```python
from build123d import *

# Parameters (mm, degrees)
SKETCH1_W           = 50
SKETCH1_H           = 52
BOSS_EXTRUDE1_DEPTH = 82.5
SKETCH2_R           = 15
CUT_EXTRUDE1_DEPTH  = 80
SKETCH3_R           = 5.25
SKETCH3_R_2         = 1.75
CUT_EXTRUDE2_DEPTH  = 91.040268769
SKETCH4_R           = 1.7
CUT_EXTRUDE4_DEPTH  = 100.911210582
SKETCH6_W           = 27.5
SKETCH6_H           = 52
CUT_EXTRUDE5_DEPTH  = 100.911210582
CUT_EXTRUDE6_DEPTH  = 100.911210582
CUT_EXTRUDE7_DEPTH  = 101.673978763
FILLET1_R           = 3


with BuildPart() as part:
    # Sketch1 → Boss-Extrude1 (new body)
    with BuildSketch(Plane.XY):
        Rectangle(SKETCH1_W, SKETCH1_H)
    extrude(amount=BOSS_EXTRUDE1_DEPTH)

    # Sketch2 → Cut-Extrude1 (cut)
    with BuildSketch(Plane(origin=(0, 0, 0), x_dir=(-1, 0, 0), z_dir=(0, 0, -1))):
        Circle(SKETCH2_R)
    extrude(amount=-CUT_EXTRUDE1_DEPTH, mode=Mode.SUBTRACT)

    # Sketch3 → Cut-Extrude2 (cut, through all)
    with BuildSketch(Plane.XY.offset(82.5)):
        Circle(SKETCH3_R)
        with Locations((-8, 0)):
            Circle(SKETCH3_R_2)
        with Locations(Location((8, 0, 0), (0, 0, 180))):
            Circle(SKETCH3_R_2)
    extrude(amount=-CUT_EXTRUDE2_DEPTH, mode=Mode.SUBTRACT)

    # Sketch4 → Cut-Extrude4 (cut, through all)
    with BuildSketch(Plane(origin=(25, 0, 0), x_dir=(0, 0, -1), z_dir=(1, 0, 0))):
        with Locations(Location((-57.5, 20, 0), (0, 0, 90))):
            Circle(SKETCH4_R)
        with Locations(Location((-57.5, -20, 0), (0, 0, 270))):
            Circle(SKETCH4_R)
    extrude(amount=-CUT_EXTRUDE4_DEPTH, mode=Mode.SUBTRACT)

    # Sketch6 → Cut-Extrude5 (cut, through all)
    with BuildSketch(Plane(origin=(25, 0, 0), x_dir=(0, 0, -1), z_dir=(1, 0, 0))):
        with Locations((-13.75, 0)):
            Rectangle(SKETCH6_W, SKETCH6_H)
    extrude(amount=-CUT_EXTRUDE5_DEPTH, mode=Mode.SUBTRACT)

    # Sketch9 → Cut-Extrude6 (cut, through all)
    with BuildSketch(Plane(origin=(25, 0, 0), x_dir=(0, 0, -1), z_dir=(1, 0, 0))):
        Polygon((-82.5, 26), (-82.5, 16), (-67.5, 26), align=None)
        Polygon((-82.5, -16), (-67.5, -26), (-82.5, -26), align=None)
    extrude(amount=-CUT_EXTRUDE6_DEPTH, mode=Mode.SUBTRACT)

    # Sketch10 → Cut-Extrude7 (cut, through all)
    with BuildSketch(Plane.XZ.offset(26)):
        Polygon((15, 82.5), (25, 67.5), (25, 82.5), align=None)
        Polygon((-25, 67.5), (-25, 82.5), (-15, 82.5), align=None)
    extrude(amount=-CUT_EXTRUDE7_DEPTH, mode=Mode.SUBTRACT)

    # Fillet1
    # the kernel refuses this fillet: 3 mm, written as the material it takes off along each edge
    with BuildSketch(Plane(origin=(-22, 23, 30.5), x_dir=(-1, 0, 0), z_dir=(0, 1, 0))) as fillet1_piece_1_section:
        Polygon((0, 0), (FILLET1_R, 0), (FILLET1_R, -FILLET1_R), (0, -FILLET1_R), align=None)
    fillet1_piece_1 = extrude(amount=FILLET1_R, mode=Mode.PRIVATE)
    fillet1_piece_1 = fillet1_piece_1 - Plane(origin=(-22, 23, 30.5), x_dir=(0.7071067811865475, 0, 0.7071067811865475), z_dir=(0, 1, 0)) * Sphere(FILLET1_R, mode=Mode.PRIVATE)
    add(fillet1_piece_1, mode=Mode.SUBTRACT)
    with BuildSketch(Plane(origin=(-22, -23, 30.5), x_dir=(0, 0, -1), z_dir=(-1, 0, 0))) as fillet1_piece_2_section:
        Polygon((0, 0), (FILLET1_R, 0), (FILLET1_R, FILLET1_R), (0, FILLET1_R), align=None)
    fillet1_piece_2 = extrude(amount=FILLET1_R, mode=Mode.PRIVATE)
    fillet1_piece_2 = fillet1_piece_2 - Plane(origin=(-22, -23, 30.5), x_dir=(0, 0.7071067811865475, 0.7071067811865475), z_dir=(-1, 0, 0)) * Sphere(FILLET1_R, mode=Mode.PRIVATE)
    add(fillet1_piece_2, mode=Mode.SUBTRACT)
    with BuildSketch(Plane(origin=(22, -23, 30.5), x_dir=(0, 0, -1), z_dir=(1, 0, 0))) as fillet1_piece_3_section:
        Polygon((0, 0), (FILLET1_R, 0), (FILLET1_R, -FILLET1_R), (0, -FILLET1_R), align=None)
    fillet1_piece_3 = extrude(amount=FILLET1_R, mode=Mode.PRIVATE)
    fillet1_piece_3 = fillet1_piece_3 - Plane(origin=(22, -23, 30.5), x_dir=(0, 0.7071067811865475, 0.7071067811865475), z_dir=(1, 0, 0)) * Sphere(FILLET1_R, mode=Mode.PRIVATE)
    add(fillet1_piece_3, mode=Mode.SUBTRACT)
    with BuildSketch(Plane(origin=(22, 23, 30.5), x_dir=(1, 0, 0), z_dir=(0, 1, 0))) as fillet1_piece_4_section:
        Polygon((0, 0), (FILLET1_R, 0), (FILLET1_R, FILLET1_R), (0, FILLET1_R), align=None)
    fillet1_piece_4 = extrude(amount=FILLET1_R, mode=Mode.PRIVATE)
    fillet1_piece_4 = fillet1_piece_4 - Plane(origin=(22, 23, 30.5), x_dir=(-0.7071067811865475, 0, 0.7071067811865475), z_dir=(0, 1, 0)) * Sphere(FILLET1_R, mode=Mode.PRIVATE)
    add(fillet1_piece_4, mode=Mode.SUBTRACT)
    with BuildSketch(Plane(origin=(12.352941176, -13.352941176, 86.470588235), x_dir=(0.26906911759852636, 0.8744746321952062, -0.40360367639778677), z_dir=(0.4850712500726659, -0.4850712500726661, -0.7276068751089989)), Plane(origin=(12.352941176, 13.352941176, 86.470588235), x_dir=(-0.8744746321952062, 0.26906911759852264, -0.4036036763977888), z_dir=(0.4850712500726658, 0.48507125007266627, -0.7276068751089988))) as fillet1_piece_5:
        with BuildLine():
            CenterArc((FILLET1_R * 0.727606875109, -FILLET1_R), FILLET1_R, 90, 72.079786861)
            Line((-FILLET1_R * 0.223879038495, -FILLET1_R * 0.692307692308), (0, 0))
            Line((0, 0), (FILLET1_R * 0.727606875109, 0))
        make_face()
    extrude(amount=31.529631255, mode=Mode.SUBTRACT)
    with BuildSketch(Plane(origin=(-12.352941176, -13.352941176, 86.470588235), x_dir=(-0.26906911759852215, 0.8744746321952062, -0.4036036763977897), z_dir=(-0.485071250072666, -0.48507125007266627, -0.7276068751089988)), Plane(origin=(-12.352941176, 13.352941176, 86.470588235), x_dir=(0.8744746321952063, 0.2690691175985245, -0.40360367639778794), z_dir=(-0.485071250072666, 0.48507125007266605, -0.7276068751089988))) as fillet1_piece_6:
        with BuildLine():
            CenterArc((FILLET1_R * 0.727606875109, FILLET1_R), FILLET1_R, 197.920213139, 72.079786861)
            Line((-FILLET1_R * 0.223879038495, FILLET1_R * 0.692307692308), (0, 0))
            Line((0, 0), (FILLET1_R * 0.727606875109, 0))
        make_face()
    extrude(amount=31.529631255, mode=Mode.SUBTRACT)
    with BuildSketch(Plane(origin=(-25, 23, 27.5), x_dir=(0, 0, 1), z_dir=(0, -1, 0)), Plane(origin=(25, -23, 27.5), x_dir=(0, 0, 1), z_dir=(0, 1, 0))) as fillet1_piece_7:
        with BuildLine():
            CenterArc((FILLET1_R, -FILLET1_R), FILLET1_R, 90, 90)
            Line((0, -FILLET1_R), (0, 0))
            Line((0, 0), (FILLET1_R, 0))
        make_face()
    extrude(amount=46, mode=Mode.SUBTRACT)
    with BuildSketch(Plane(origin=(22, -26, 27.5), x_dir=(0, 1, 0), z_dir=(-1, 0, 0)), Plane(origin=(22, 26, 27.5), x_dir=(0, 0, 1), z_dir=(-1, 0, 0))) as fillet1_piece_8:
        with BuildLine():
            CenterArc((FILLET1_R, -FILLET1_R), FILLET1_R, 90, 90)
            Line((0, -FILLET1_R), (0, 0))
            Line((0, 0), (FILLET1_R, 0))
        make_face()
    extrude(amount=44, mode=Mode.SUBTRACT)
    with BuildSketch(Plane(origin=(0, 0, 27.5), x_dir=(-1, 0, 0), z_dir=(0, -1, 0))) as fillet1_piece_9:
        with BuildLine():
            CenterArc((15 + FILLET1_R, -FILLET1_R), FILLET1_R, 90, 90)
            Line((15, -FILLET1_R), (15, 0))
            Line((15, 0), (15 + FILLET1_R, 0))
        make_face()
    revolve(axis=Axis((0, 0, 27.5), (0, 0, -1)), mode=Mode.SUBTRACT)
    with BuildSketch(Plane(origin=(-25, -26, 30.5), x_dir=(0, 1, 0), z_dir=(0, 0, 1)), Plane(origin=(-25, 26, 30.5), x_dir=(1, 0, 0), z_dir=(0, 0, 1))) as fillet1_piece_10:
        with BuildLine():
            CenterArc((FILLET1_R, -FILLET1_R), FILLET1_R, 90, 90)
            Line((0, -FILLET1_R), (0, 0))
            Line((0, 0), (FILLET1_R, 0))
        make_face()
    extrude(amount=44.5, mode=Mode.SUBTRACT)
    with BuildSketch(Plane(origin=(25, -26, 30.5), x_dir=(0, 1, 0), z_dir=(0, 0, 1)), Plane(origin=(25, 26, 30.5), x_dir=(-1, 0, 0), z_dir=(0, 0, 1))) as fillet1_piece_11:
        with BuildLine():
            CenterArc((FILLET1_R, FILLET1_R), FILLET1_R, 180, 90)
            Line((0, FILLET1_R), (0, 0))
            Line((0, 0), (FILLET1_R, 0))
        make_face()
    extrude(amount=44.5, mode=Mode.SUBTRACT)


solid = part.part
```
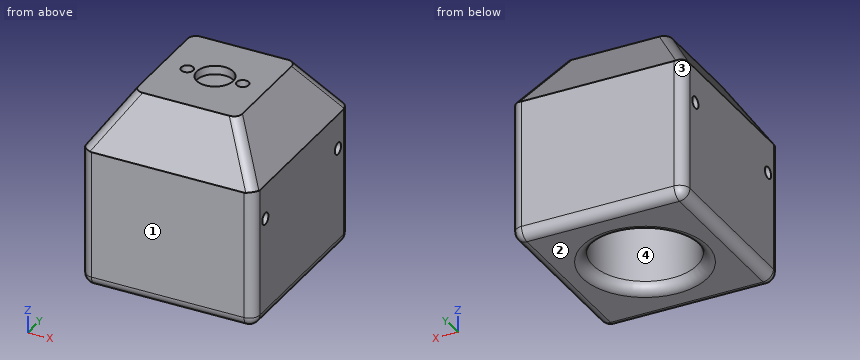
The listing builds one solid part. Answer for the finished solid, in the listing's coordinates (mm). Face numbers are marked on the shaded views. Coordinates: 2 decimals unless noted, no trailing zeros. Write each loop counter-clockwise with the first axis right and the second up, starting at its lowest first coordinate (ties: lowest second). Pieces come first, ordered by that corner, then holes.
Q1. Given P1, Ø24, axis at x = 5, y = 1, coming from the -Z side; P2, Ø5.5, axis at x = 8, y = 0, coming from the -Z side, each flat-ended and moving along its own axis, determine where each tip first touches the part or whether it passes through.
Returned:
P1: stops at z = 27.64
P2: stops at z = 80
Q2. The mould has two halves that part along Y. Classify the marked faces 1, 2, 3 and 4: released by +Y, released by -Y, zero draft, split by the parting line, or undercut.
Returned:
face 1: released by -Y
face 2: zero draft
face 3: released by +Y
face 4: undercut
Q3. Section D-D, the plane z = 41 is taken. Write down the section's boundary in (x, y).
Returned:
outline: (-25, -23) arc R3 ccw to (-22, -26) - (22, -26) arc R3 ccw to (25, -23) - (25, 23) arc R3 ccw to (22, 26) - (-22, 26) arc R3 ccw to (-25, 23) - close; hole circle Ø30 at (0, 0)
Q4. Section C-C, the plane y = 0 is taken. Write down the section's boundary in (x, z).
Returned:
outline: (-25, 30.5) arc R3 ccw to (-22, 27.5) - (-18, 27.5) arc R3 ccw to (-15, 30.5) - (-15, 80) - (-9.75, 80) - (-9.75, 82.5) - (-15, 82.5) - (-25, 67.5) - close; (-6.25, 80) - (-5.25, 80) - (-5.25, 82.5) - (-6.25, 82.5) - close; (5.25, 80) - (6.25, 80) - (6.25, 82.5) - (5.25, 82.5) - close; (9.75, 80) - (15, 80) - (15, 30.5) arc R3 ccw to (18, 27.5) - (22, 27.5) arc R3 ccw to (25, 30.5) - (25, 67.5) - (15, 82.5) - (9.75, 82.5) - close
Q5. Section B-B, the plane z = 57.5 is taken. Write down the section's boundary in (x, y).
Returned:
outline: (-25, -23) arc R3 ccw to (-22, -26) - (22, -26) arc R3 ccw to (25, -23) - (25, -21.7) - (-25, -21.7) - close; (-25, -18.3) - (25, -18.3) - (25, 18.3) - (-25, 18.3) - close; (-25, 21.7) - (25, 21.7) - (25, 23) arc R3 ccw to (22, 26) - (-22, 26) arc R3 ccw to (-25, 23) - close; hole circle Ø30 at (0, 0)
Q6. Find the intervals of material crossed by line 1 along Y through (x, z) = (-21.5, 58.5); line 2 along Z through (x, y) = (-3.5, 11.5); line 3 along X through (y, z) = (-4, 35), in increasing order.
Returned:
line 1: y = -26 to -21.37, -18.63 to 18.63, 21.37 to 26
line 2: z = 80 to 82.5
line 3: x = -25 to -14.46, 14.46 to 25
Q7. Section A-A, the plane x = 0 is taken. Write down the section's boundary in (y, z).
Returned:
outline: (-26, 30.5) arc R3 ccw to (-23, 27.5) - (-18, 27.5) arc R3 ccw to (-15, 30.5) - (-15, 80) - (-5.25, 80) - (-5.25, 82.5) - (-16, 82.5) - (-26, 67.5) - close; (5.25, 80) - (15, 80) - (15, 30.5) arc R3 ccw to (18, 27.5) - (23, 27.5) arc R3 ccw to (26, 30.5) - (26, 67.5) - (16, 82.5) - (5.25, 82.5) - close; hole circle Ø3.4 at (-20, 57.5); hole circle Ø3.4 at (20, 57.5)
